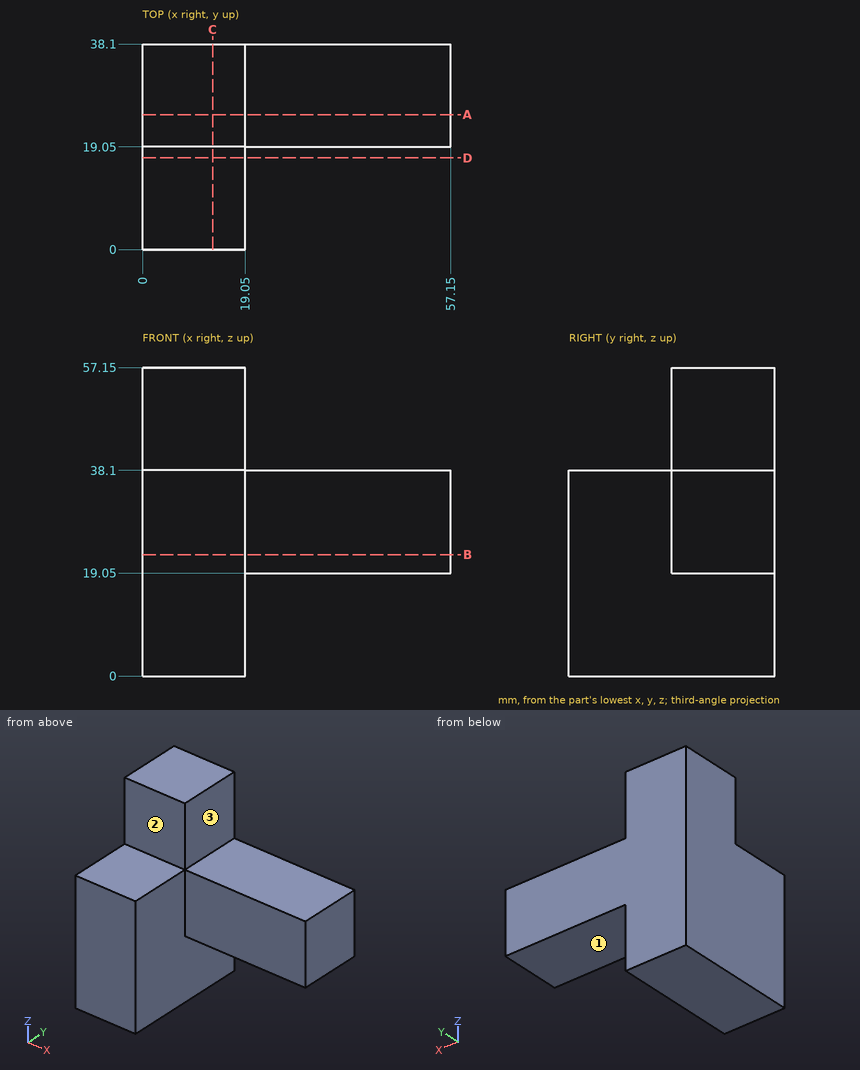
The figure shows three views and two pictorial views of one solid part (mm, origin at its lowest corner). Answer the questions. A direction names the side the tool comes from. Coordinates: 2 decimals unless noted, no trailing zeros. Loops run counter-clockwise (first coordinate to the right, second up) from the corner with the lowest first, then second, coordinate; pieces in that order, holes last. Notation, with made-up numbers: (-21, 20) -> (0, 20) arc R24 cw to (0, 33) -> close; hole circle Ø5 at (-25.75, -24.75). An arc over 180 degrees is marked (long way). Use one line per item in the form item = value. Start each with the question number.
Item 1: Consider L1, parallel to Z at x = 53, y = 28.5; L2, parallel to X at y = 31, z = 3. Determine where each line is inside the solid, lowest interval first. Write a range as [from, to].
Item 2: The part is cut by section B-B on z = 22.5. Determine the outline of the cut face in (x, y).
Item 3: A tool of negligible diameter and unlimited length cuts with its end or side. For the marked faces 1, 2 and 3, from which of +Z, -Z, +X, -X, +Y, -Y can it reach the whole face along a straight path? Write none if from no direction.
Item 4: Flat-ended cylindrical pins translate along their axes: pin 1 Ø21 at (x, y) = (6, 8.5) entering from +Z; pin 2 Ø9.5 at (x, z) = (5, 51.5) entering from -Y; pin 3 Ø21 at (x, z) = (44.5, 31) entering from -Y. Find the tip coordinate at first contact, or state that the pin passes through.
Item 5: The part is cut by section D-D on y = 17. Determine the outline of the cut face in (x, z), then the cut area to 3 significant figures.
Item 6: The part is cut by section C-C on x = 13. Determine the outline of the cut face in (y, z).
Item 7: The part is cut by section A-A on y = 25. Determine the outline of the cut face in (x, z).
Answer key:
q1.L1 = [19.05, 38.1]
q1.L2 = [0, 19.05]
q2.outline = (0, 0) -> (19.05, 0) -> (19.05, 19.05) -> (57.15, 19.05) -> (57.15, 38.1) -> (0, 38.1) -> close
q3.face_1 = -Z, +X, +Y, -Y
q3.face_2 = +Z, +X, -X, -Y
q3.face_3 = +Z, +X, +Y, -Y
q4.pin_1 = 38.1
q4.pin_2 = 19.05
q4.pin_3 = 19.05
q5.outline = (0, 0) -> (19.05, 0) -> (19.05, 38.1) -> (0, 38.1) -> close
q5.area = 726 mm2
q6.outline = (0, 0) -> (38.1, 0) -> (38.1, 57.15) -> (19.05, 57.15) -> (19.05, 38.1) -> (0, 38.1) -> close
q7.outline = (0, 0) -> (19.05, 0) -> (19.05, 19.05) -> (57.15, 19.05) -> (57.15, 38.1) -> (19.05, 38.1) -> (19.05, 57.15) -> (0, 57.15) -> close
